from build123d import *

# Parameters (mm, degrees)
SALIENTE_EXTRUIR1_DEPTH = 4
CROQUIS3_R              = 3
CORTAR_EXTRUIR1_DEPTH   = 5


with BuildPart() as part:
    # Croquis2 → Saliente-Extruir1 (new body)
    with BuildSketch(Plane.XY):
        Polygon((5, 0), (2.5, 4.330127019), (-2.5, 4.330127019), (-5, 0), (-2.5, -4.330127019), (2.5, -4.330127019), align=None)
    extrude(amount=SALIENTE_EXTRUIR1_DEPTH)

    # Croquis3 → Cortar-Extruir1 (cut, through all)
    with BuildSketch(Plane(origin=(0, 0, 0), x_dir=(-1, 0, 0), z_dir=(0, 0, -1))):
        Circle(CROQUIS3_R)
    extrude(amount=-CORTAR_EXTRUIR1_DEPTH, mode=Mode.SUBTRACT)


solid = part.part
For this review, take the finished solid that the model builds, in its own axes (mm). Give positions to 0.01 mm unless a question says otherwise; leave off trailing zeros. Write each loop counter-clockwise with the first axis right and the second up, starting at its lowest first coordinate (ties: lowest second). Pieces come first, ordered by that corner, then holes. Notation, with made-up numbers: (64.25, 58) -> (80.25, 58) arc R15 ccw to (80.25, 68) -> close; hole circle Ø8 at (22, -11). An arc over 180 degrees is marked (long way). Use CSV: the item, a comma, the result in double quotes.
Q1. To check wall thickness, follow probe 1 along Y at (x, z) = (0, 2.4); probe 2 along X at (y, z) = (2, 3.15); probe 3 along Y at (x, z) = (-2, 0.35). State the ranges of each line that lie inside material, in increasing order. Write a range as [from, to].
Conclusion:
probe 1,"[-4.33, -3], [3, 4.33]"
probe 2,"[-3.85, -2.24], [2.24, 3.85]"
probe 3,"[-4.33, -2.24], [2.24, 4.33]"
Q2. Take a section at A-A, the plane x = 0. Write out the cut boundary in (y, z).
Conclusion:
outline,"(-4.33, 0) -> (-3, 0) -> (-3, 4) -> (-4.33, 4) -> close; (3, 0) -> (4.33, 0) -> (4.33, 4) -> (3, 4) -> close"
Q3. For P1, Ø5, axis at x = -3.5, y = 2, coming from the -Z side; P2, Ø1.5, axis at x = -4, z = 2, coming from the +Y side; P3, Ø1.5, axis at y = -3.5, z = 1.5, coming from the +X side, all flat-tipped, find the tip position at first contact; note any pin that passes through.
Conclusion:
P1,"z = 0"
P2,"y = 3.03"
P3,"x = 3.41"
Q4. Take a section at D-D, the plane x = 4.5. Write out the cut boundary in (y, z), then the cut area to 3 significant figures.
Conclusion:
outline,"(-0.87, 0) -> (0.87, 0) -> (0.87, 4) -> (-0.87, 4) -> close"
area,"6.93 mm2"
Q5. Take a section at B-B, the plane z = 1.6. Write out the cut boundary in (x, y), then the cut area to 3 significant figures.
Conclusion:
outline,"(-5, 0) -> (-2.5, -4.33) -> (2.5, -4.33) -> (5, 0) -> (2.5, 4.33) -> (-2.5, 4.33) -> close; hole circle Ø6 at (0, 0)"
area,"36.7 mm2"
Q6. Mouldability with a two-part tool opening along Y and no side actions: class faces 1 (the face through (1, 3, 4)), 2 (the face through (3, 0, 2)), 3 (the face through (-3.73, 2.2, 1.97)) as pulls with the +Y half, pulls with the -Y half, needs draft (parallel to the pull), parting line crosses it, or undercut.
Conclusion:
face 1,"needs draft"
face 2,"undercut"
face 3,"pulls with the +Y half"
Q7. Take a section at C-C, the plane y = 0.75. Write out the cut boundary in (x, z).
Conclusion:
outline,"(-4.57, 0) -> (-2.9, 0) -> (-2.9, 4) -> (-4.57, 4) -> close; (2.9, 0) -> (4.57, 0) -> (4.57, 4) -> (2.9, 4) -> close"
